```python
from build123d import *

# Parameters (mm, degrees)
F1_DEPTH = 400
F2_W     = 500
F2_H     = 700
F3_DEPTH = 840
F4_W     = 500
F4_H     = 700
F5_DEPTH = 124


with BuildPart() as f1:
    # F0 (on Front) → F1 (new body, symmetric)
    with BuildSketch(Plane.XZ):
        Polygon((-250, 224.901706), (0, 224.901706), (250, 224.901706), (250, 0), (400, 0), (400, 858.125869), (850, 1050), (850, 1200), (0, 1200), (-850, 1200), (-850, 1050), (-400, 858.125869), (-400, 0), (-250, 0), align=None)
    extrude(amount=F1_DEPTH, both=True)

    # F2 (on face) → F3 (cut)
    with BuildSketch(Plane.XY.offset(1200)):
        Rectangle(F2_W, F2_H)
    extrude(amount=-F3_DEPTH, mode=Mode.SUBTRACT)

    # F4 (on face) → F5 (cut)
    with BuildSketch(Plane.XY.offset(1200)):
        with Locations((-550, 0)):
            Rectangle(F4_W, F4_H)
        with Locations((550, 0)):
            Rectangle(F4_W, F4_H)
    extrude(amount=-F5_DEPTH, mode=Mode.SUBTRACT)


solid = f1.part
```
Source: CAD feature listing. Evaluate the final solid. Frame: model axes, mm. A direction names the side the tool comes from. Coordinates: 2 decimals unless noted, no trailing zeros. Loops run counter-clockwise (first coordinate to the right, second up) from the corner with the lowest first, then second, coordinate; pieces in that order, holes last. Notation, with made-up numbers: M -23.75,-38.5 L -13.75,-38.5 A16 cw -13.75,-33.5 Z; hole C 2,14 d11. An arc over 180 degrees is marked long. Put each result on its own line as item: value. Start each with the question number.
1) Cut plane B-B on x = 72.5. Return the cut outline in (y, z), then the cut area to 3 significant figures.
2) Cut plane C-C on z = 154. Return the cut outline in (x, y), then the cut area to 3 significant figures.
3) Reachability of faces 4 (the face through (-400, -6, 435)), 5 (the face through (850, -6, 1124)), 6 (the face through (-554, -350, 1139)), 7 (the face through (250, -6, 114)), 8 (the face through (-850, -6, 1126)) from +Z, -Z, +X, -X, +Y, -Y: full face, straight path, thin tool, end or side. Return the list, or none.
4) Pull-direction query (Y, two-part tool) for faces 1 (the face through (300, -5, 1139)), 2 (the face through (-12, -400, 742)), 3 (the face through (-3, -6, 224.902)); classes: pulls with the +Y half, pulls with the -Y half, needs draft (parallel to the pull), parting line crosses it, or undercut.
5) Cut plane D-D on y = 251. Return the cut outline in (x, z).
6) Ray query, L1, parallel to X at y = -345, z = 131; L2, parallel to X at y = 262, z = 1070; L3, parallel to X at y = 329.5, z = 1130.5. Return the intervals inside material, ascending. Write a range as from..to.
7) Contact query for flat-ended pins moving along their axis: pin 1 Ø1.5 at (y, z) = (-41.5, 220) entering from -X; pin 2 Ø3 at (y, z) = (314.5, 516.5) entering from +X; pin 3 Ø12 at (y, z) = (21.5, 880.5) entering from -X. Output: stop coordinate, or through.
8) Cut plane A-A on z = 1117. Return the cut outline in (x, y), then the cut area to 3 significant figures.
The answers:
1. outline: M -400,224.9 L 400,224.9 L 400,1200 L 350,1200 L 350,360 L -350,360 L -350,1200 L -400,1200 Z
1. area: 192,000 mm²
2. outline: M -400,-400 L -250,-400 L -250,400 L -400,400 Z; M 250,-400 L 400,-400 L 400,400 L 250,400 Z
2. area: 240,000 mm²
3. face 4: -Z, -X, +Y, -Y
3. face 5: +Z, -Z, +X, +Y, -Y
3. face 6: +Z
3. face 7: -Z, +Y, -Y
3. face 8: +Z, -Z, -X, +Y, -Y
4. face 1: undercut
4. face 2: pulls with the -Y half
4. face 3: needs draft
5. outline: M -850,1050 L -400,858.13 L -400,0 L -250,0 L -250,224.9 L 250,224.9 L 250,0 L 400,0 L 400,858.13 L 850,1050 L 850,1200 L 800,1200 L 800,1076 L 300,1076 L 300,1200 L 250,1200 L 250,360 L -250,360 L -250,1200 L -300,1200 L -300,1076 L -800,1076 L -800,1200 L -850,1200 Z
6. L1: x = -400..-250, 250..400
6. L2: x = -850..-250, 250..850
6. L3: x = -850..-800, -300..-250, 250..300, 800..850
7. pin 1: stops at x = -400
7. pin 2: stops at x = 400
7. pin 3: stops at x = -466.55
8. outline: M -850,-400 L 850,-400 L 850,400 L -850,400 Z; hole M -800,-350 L -300,-350 L -300,350 L -800,350 Z; hole M -250,-350 L 250,-350 L 250,350 L -250,350 Z; hole M 300,-350 L 800,-350 L 800,350 L 300,350 Z
8. area: 310,000 mm²
